from build123d import *

# Parameters (mm, degrees)
BOSS_EXTRUDE1_DEPTH      = 2.5
EXTRUDE_THIN1_DEPTH      = 0.5
EXTRUDE_THIN1_DEPTH_BACK = 0.5
CHAMFER1_SIZE            = 0.4


with BuildPart() as part:
    # Sketch1 → Boss-Extrude1 (new body)
    with BuildSketch(Plane(origin=(0, 0, 0), x_dir=(-1, 0, 0), z_dir=(0, 1, 0))):
        Polygon((-1.02, 1.27), (1.02, 1.27), (1.27, 1.02), (1.27, -1.02), (1.02, -1.27), (-1.02, -1.27), (-1.27, -1.02), (-1.27, 1.02), align=None)
    extrude(amount=BOSS_EXTRUDE1_DEPTH)

    # Sketch2 → Extrude-Thin1 (add, two sides)
    with BuildSketch(Plane(origin=(0, 0, 0), x_dir=(0, 0, -1), z_dir=(1, 0, 0))) as extrude_thin1_sk:
        with BuildLine():
            Line((0.5, -2.5), (0.5, 0))
            Line((0.5, 0), (0.5, 4))
            ThreePointArc((0.5, 4), (0.646446609, 4.353553391), (1, 4.5))
            Line((1, 4.5), (8, 4.5))
            Line((8, 4.5), (8, 5.5))
            Line((8, 5.5), (1, 5.5))
            ThreePointArc((1, 5.5), (-0.060660172, 5.060660172), (-0.5, 4))
            Line((-0.5, 4), (-0.5, 0))
            Line((-0.5, 0), (-0.5, -2.5))
            Line((-0.5, -2.5), (0.5, -2.5))
        make_face()
    extrude(amount=EXTRUDE_THIN1_DEPTH)
    extrude(extrude_thin1_sk.sketch, amount=-EXTRUDE_THIN1_DEPTH_BACK)

    # Chamfer1
    chamfer1_edges = [part.edges().sort_by_distance(p)[0] for p in [
        (-0.5, 5, -8),
        (0, 4.5, -8),
        (0, -2.5, -0.5),
        (0.5, -2.5, 0),
        (0, -2.5, 0.5),
        (0, 5.5, -8),
        (0.5, 5, -8),
        (-0.5, -2.5, 0),
    ]]
    chamfer(chamfer1_edges, length=CHAMFER1_SIZE)


solid = part.part
Geometry: final body of the model. Coordinates: model frame, mm. A direction names the side the tool comes from. Give positions to 0.01 mm unless a question says otherwise; leave off trailing zeros. Loops run counter-clockwise (first coordinate to the right, second up) from the corner with the lowest first, then second, coordinate; pieces in that order, holes last. Notation, with made-up numbers: (27, -3.75) -> (82, -3.75) arc R25 cw to (82, 21.25) -> close; hole circle Ø8 at (14, -12). An arc over 180 degrees is marked (long way). Put each result on its own line as item: value.
1. Cut plane A-A (y = 0.5). Return the cut outline in (x, z).
Taken from the geometry:
outline: (-1.27, -1.02) -> (-1.02, -1.27) -> (1.02, -1.27) -> (1.27, -1.02) -> (1.27, 1.02) -> (1.02, 1.27) -> (-1.02, 1.27) -> (-1.27, 1.02) -> close
2. Ray query, line 1 along Z through (x, y) = (0.55, 2); line 2 along Y through (x, z) = (-0.45, -2.5); line 3 along X through (y, z) = (5, -3). Return the intervals inside material, ascending. Write a range as [from, to].
Taken from the geometry:
line 1: z = [-1.27, 1.27]
line 2: y = [4.5, 5.5]
line 3: x = [-0.5, 0.5]
3. Cut plane B-B (x = -0.25). Return the cut outline in (y, z).
Taken from the geometry:
outline: (-2.35, -0.25) -> (-2.1, -0.5) -> (0, -0.5) -> (0, -1.27) -> (2.5, -1.27) -> (2.5, -0.5) -> (4, -0.5) arc R0.5 cw to (4.5, -1) -> (4.5, -7.6) -> (4.75, -7.85) -> (5.25, -7.85) -> (5.5, -7.6) -> (5.5, -1) arc R1.5 ccw to (4, 0.5) -> (2.5, 0.5) -> (2.5, 1.27) -> (0, 1.27) -> (0, 0.5) -> (-2.1, 0.5) -> (-2.35, 0.25) -> close
4. Set-up query: faces 1 (the flat face through (-0.5, 5, -3)), 2 (the flat face through (1, 2.5, 0)), 3 (the flat face through (0.5, -1, 0)). Return all of +Z, -Z, +X, -X, +Y, -Y with unobstructed straight access to the full face (end or side cutting, diameter ignored); none if empty.
Taken from the geometry:
face 1: +Z, -Z, -X, +Y
face 2: none
face 3: +Z, -Z, +X, -Y
5. Pin query (flat end, axial travel): P1, Ø1.5, axis at y = -1, z = -1, coming from the +X side; P2, Ø0.8, axis at x = 0, z = 0, coming from the +Y side; P3, Ø3.5, axis at y = 4.5, z = -5, coming from the -X side; P4, Ø2, axis at y = 0.5, z = -2.5, coming from the +X side. Return the tip coordinate at first contact, or that it passes through.
Taken from the geometry:
P1: stops at x = 0.5
P2: stops at y = 5.37
P3: stops at x = -0.5
P4: passes through
6. Cut plane D-D (x = 0.3). Return the cut outline in (y, z), plus the area to 3 significant figures.
Taken from the geometry:
outline: (-2.3, -0.3) -> (-2.1, -0.5) -> (0, -0.5) -> (0, -1.27) -> (2.5, -1.27) -> (2.5, -0.5) -> (4, -0.5) arc R0.5 cw to (4.5, -1) -> (4.5, -7.6) -> (4.7, -7.8) -> (5.3, -7.8) -> (5.5, -7.6) -> (5.5, -1) arc R1.5 ccw to (4, 0.5) -> (2.5, 0.5) -> (2.5, 1.27) -> (0, 1.27) -> (0, 0.5) -> (-2.1, 0.5) -> (-2.3, 0.3) -> close
area: 18.4 mm2
7. Cut plane C-C (z = -1.5). Return the cut outline in (x, y), plus the area to 3 significant figures.
Taken from the geometry:
outline: (-0.5, 4.5) -> (0.5, 4.5) -> (0.5, 5.5) -> (-0.5, 5.5) -> close
area: 1.00 mm2
